Check sheet for the drawn part. Datum: minimum x, y, z corner. Units: mm. A direction names the side the tool comes from. Give positions to 0.01 mm unless a question says otherwise; leave off trailing zeros. Loops run counter-clockwise (first coordinate to the right, second up) from the corner with the lowest first, then second, coordinate; pieces in that order, holes last.
1. Cross-section at A-A, the plane y = 12.7. State how many separate pieces and enclosed holes the cut face has, plus the area to 3 significant figures.
2. Cross-section at D-D, the plane z = 19.05. Record the cut outline in (x, y) (1 decimal).
3. Release check for a two-part mould opening along X. For the marked faces 1, 2 and 3 record: +X half, -X half, draft (parallel to the pull), parting line (faces both ways), or undercut.
4. Go/stop test with flat-tipped pins: pin 1 Ø8.5 at (x, y) = (12.7, 12.7) entering from -Z; pin 2 Ø1.5 at (x, y) = (7, 19.5) entering from +Z; pin 3 Ø5 at (x, z) = (6, 15.5) entering from -Y. Record where each tip stops, or that it passes through.
5. Tool access check on the marked faces 4 and 5. Record the directions out of +Z, -Z, +X, -X, +Y, -Y that give a thin tool (end or side, any length) a straight path to the whole face; none if there is none.
6. Material ranges on L1, parallel to X at y = 22.75, z = 7.75; L2, parallel to Y at x = 12.7, z = 4.25 (1 decimal); L3, parallel to Z at x = 22.5, y = 12.75 (1 decimal), recorded low to high.
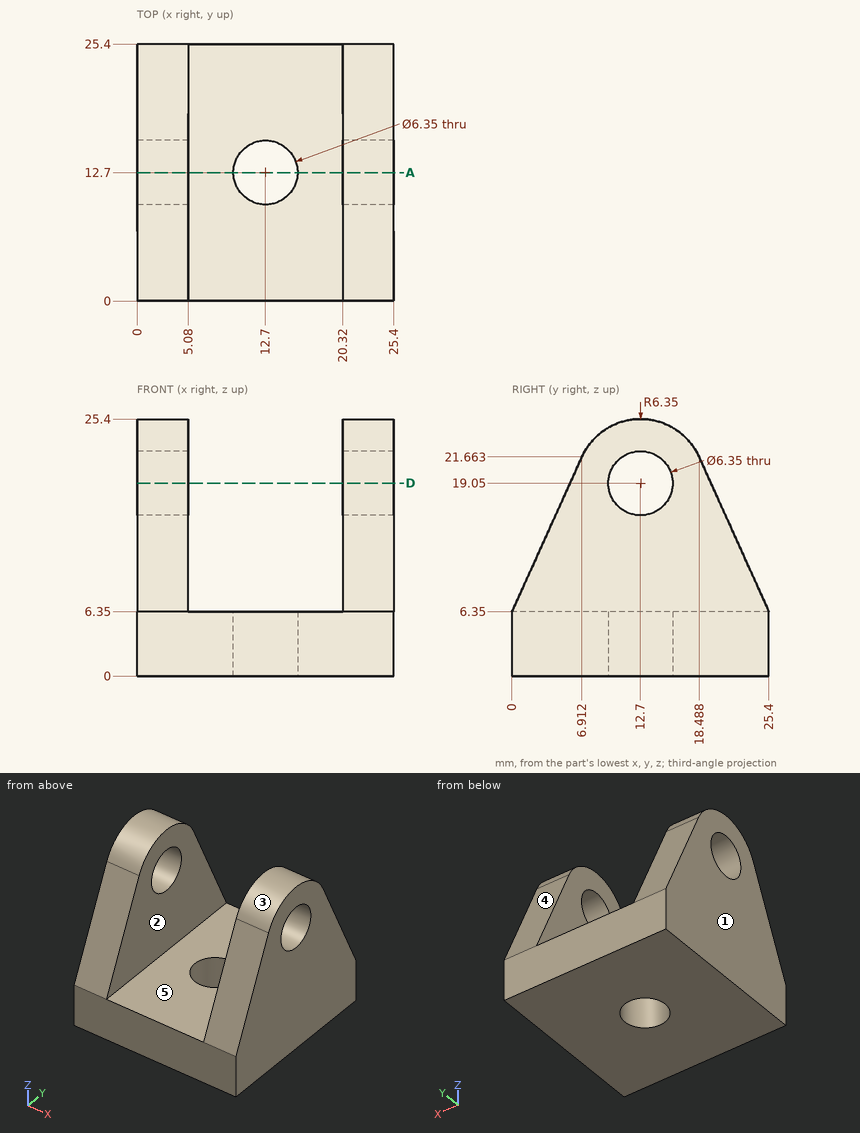
Result:
1. separate pieces: 4
1. enclosed holes: 0
1. area: 250 mm2
2. outline: (0, 5.7) - (5.1, 5.7) - (5.1, 9.5) - (0, 9.5) - close; (0, 15.9) - (5.1, 15.9) - (5.1, 19.7) - (0, 19.7) - close; (20.3, 5.7) - (25.4, 5.7) - (25.4, 9.5) - (20.3, 9.5) - close; (20.3, 15.9) - (25.4, 15.9) - (25.4, 19.7) - (20.3, 19.7) - close
3. face 1: -X half
3. face 2: undercut
3. face 3: draft
4. pin 1: stops at z = 0
4. pin 2: stops at z = 6.35
4. pin 3: stops at y = 3.08
5. face 4: +Z, +X, -X, +Y
5. face 5: +Z, +Y, -Y
6. L1: x = 0 to 5.08, 20.32 to 25.4
6. L2: y = 0 to 9.5, 15.9 to 25.4
6. L3: z = 0 to 15.9, 22.2 to 25.4
